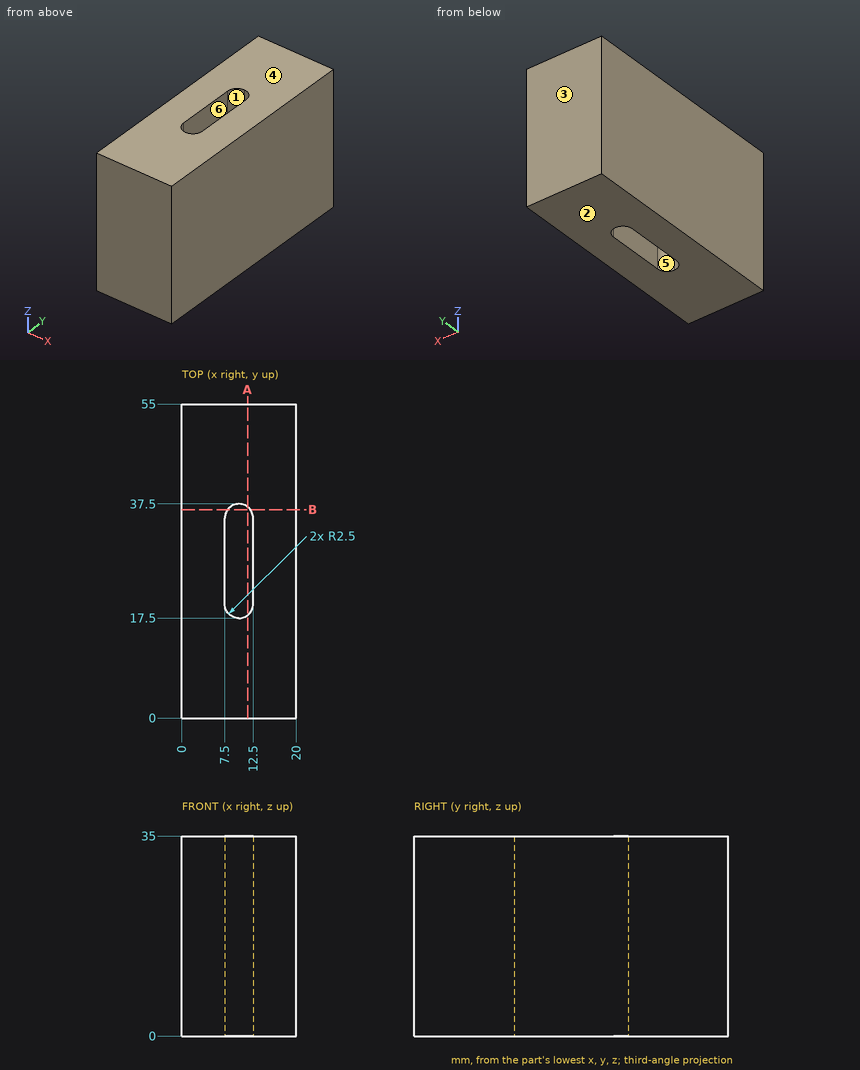
Here's the drawing with two shaded views (mm, measured from the low corner). I have some questions. A direction names the side the tool comes from. Give positions to 0.01 mm unless a question says otherwise; leave off trailing zeros. Loops run counter-clockwise (first coordinate to the right, second up) from the corner with the lowest first, then second, coordinate; pieces in that order, holes last. Notation, with made-up numbers: (-30.75, -12) - (-5.75, -12) arc R11 ccw to (-5.75, 8) - close; hole circle Ø9 at (-16.5, 24). An arc over 180 degrees is marked (long way). Answer in a Markdown table with one row per item. Add a question column.
Q1. If we section it at B-B (y = 36.5): List the corners of the cut face in (x, z) for me, plus the area to 3 significant figures.
Q2. If we section it at A-A (x = 11.5): List the corners of the cut face in (y, z) for me, plus the area to 3 significant figures.
Q3. Which directions (+Z, -Z, +X, -X, +Y, -Y) give clear straight access to the entire face, cutting with the end or side of a thin tool? Please do the marked faces 1 and 2.
Q4. Please list where these lines run through material, in increasing order: L1, parallel to X at y = 29.5, z = 24; L2, parallel to Y at x = 10.25, z = 21. Write a range as from..to.
Q5. We'd pull the mould along Y, two halves only. Please class the marked faces 3, 4, 5 and 6: +Y half, -Y half, draft (parallel to the pull), parting line (faces both ways), or undercut.
The answers:
| question | item | result |
|---|---|---|
| 1 | outline | (0, 0) - (8, 0) - (8, 35) - (0, 35) - close; (12, 0) - (20, 0) - (20, 35) - (12, 35) - close |
| 1 | area | 560 mm^2 |
| 2 | outline | (0, 0) - (18, 0) - (18, 35) - (0, 35) - close; (37, 0) - (55, 0) - (55, 35) - (37, 35) - close |
| 2 | area | 1,260 mm^2 |
| 3 | face 1 | +Z, -Z |
| 3 | face 2 | -Z, +X, -X, +Y, -Y |
| 4 | L1 | x = 0..7.5, 12.5..20 |
| 4 | L2 | y = 0..17.51, 37.49..55 |
| 5 | face 3 | +Y half |
| 5 | face 4 | draft |
| 5 | face 5 | undercut |
| 5 | face 6 | undercut |
